Model file for the job. Use its own axes, mm. A direction names the side the tool comes from. Give positions to 0.01 mm unless a question says otherwise; leave off trailing zeros. Loops run counter-clockwise (first coordinate to the right, second up) from the corner with the lowest first, then second, coordinate; pieces in that order, holes last. Notation, with made-up numbers: M -26.75,28 L 32.25,28 A13 cw 32.25,48 Z; hole C -0.5,44.5 d3. An arc over 180 degrees is marked long. Answer in a Markdown table with one row per item.
```python
from build123d import *

# Parameters (mm, degrees)
F0_R     = 2.5
F1_DEPTH = 40
F3_DEPTH = 4
F5_DEPTH = 4


with BuildPart() as f1:
    # F0 (on Top) → F1 (new body)
    with BuildSketch(Plane.XY):
        Circle(F0_R)
    extrude(amount=F1_DEPTH)

    # F2 (on face) → F3 (join)
    with BuildSketch(Plane.XY.offset(40)):
        Polygon((3, -1.732051), (3, 1.732051), (0, 3.464102), (-3, 1.732051), (-3, -1.732051), (0, -3.464102), align=None)
    extrude(amount=F3_DEPTH)

    # F4 (on face) → F5 (join)
    with BuildSketch(Plane.XY.offset(44)):
        Polygon((3.5, -2.020726), (3.5, 2.020726), (0, 4.041452), (-3.5, 2.020726), (-3.5, -2.020726), (0, -4.041452), align=None)
    extrude(amount=F5_DEPTH)


solid = f1.part
```
Q1. Saw through at D-D (y = 3). Give the cut face in (x, z).
Reported:
| item | result |
|---|---|
| outline | M -1.8,44 L -0.8,44 L -0.8,40 L 0.8,40 L 0.8,44 L 1.8,44 L 1.8,48 L -1.8,48 Z |
Q2. Drop flat-ended pins along their axis: pin 1 (4 mm diameter, centred on y = 0.5, z = 41.5, fed in from +X); pin 2 (1 mm diameter, centred on x = -2, z = 18.5, fed in from +Y); pin 3 (1.7 mm diameter, centred on y = -0.5, z = 42, fed in from -X). Give the stop position or say it passes through.
Reported:
| item | result |
|---|---|
| pin 1 | x = 3 |
| pin 2 | y = 2 |
| pin 3 | x = -3 |
Q3. Saw through at B-B (z = 43). Give the cut face in (x, y), and give its area (3 significant figures).
Reported:
| item | result |
|---|---|
| outline | M -3,-1.73 L 0,-3.46 L 3,-1.73 L 3,1.73 L 0,3.46 L -3,1.73 Z |
| area | 31.2 mm² |
Q4. Probe probe 1 along Y at (x, z) = (-1, 46); probe 2 along Z at (x, y) = (3, -2); probe 3 along Z at (x, y) = (2, -2). List the from-to ranges inside material, lowest first.
Reported:
| item | result |
|---|---|
| probe 1 | -3.46 to 3.46 |
| probe 2 | 44 to 48 |
| probe 3 | 40 to 48 |
Q5. Saw through at A-A (y = 0). Give the cut face in (x, z).
Reported:
| item | result |
|---|---|
| outline | M -3.5,44 L -3,44 L -3,40 L -2.5,40 L -2.5,0 L 2.5,0 L 2.5,40 L 3,40 L 3,44 L 3.5,44 L 3.5,48 L -3.5,48 Z |
Q6. 3-axis set-ups, long thin cutter, end or side, ignore diameter. For faces 1 (the face through (1.5, 2.6, 42)), 2 (the face through (1.5, -2.6, 42)), 3 (the face through (-1.3, -3, 44)), 4 (the face through (3, 0, 42)), 5 (the face through (-1.5, -2.6, 42)): which of +Z, -Z, +X, -X, +Y, -Y reach the whole face in a straight line?
Reported:
| item | result |
|---|---|
| face 1 | -Z, +X, +Y |
| face 2 | -Z, +X, -Y |
| face 3 | -Z |
| face 4 | -Z, +X, +Y, -Y |
| face 5 | -Z, -X, -Y |
Q7. Saw through at C-C (z = 11.5). Give the cut face in (x, y).
Reported:
| item | result |
|---|---|
| outline | C 0,0 d5 |
